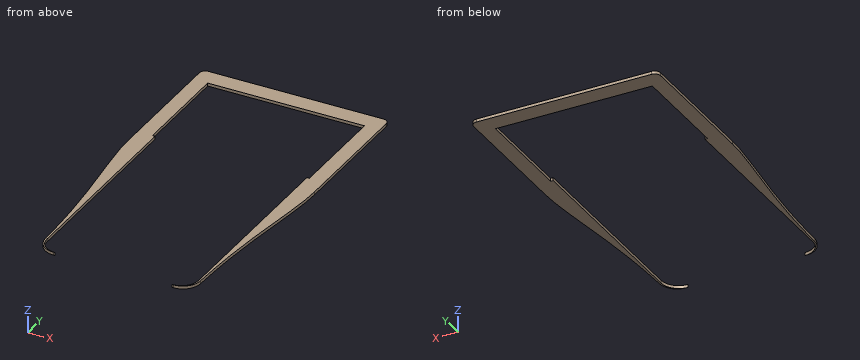
```python
from build123d import *

# Parameters (mm, degrees)
BOSS_EXTRUDE1_START = -1.5
BOSS_EXTRUDE1_DEPTH = 1.5
CUT_EXTRUDE1_DEPTH  = 14
FILLET1_R           = 8.7
FILLET2_R           = 3


# Read off the part's stored shape, not the designer's step: Boss-Extrude1
with BuildPart() as part:
    # Boss-Extrude1 outline → Boss-Extrude1 (new body)
    with BuildSketch(Plane.XY.offset(BOSS_EXTRUDE1_START)):
        with BuildLine():
            Line((101.710048323, 103.170955585), (101.710048323, 33.070955585))
            add(Edge.make_bspline(
                [(101.710048323, 33.070955585), (101.710048323, 14.099715191), (109.710048323, -16.929044415), (109.710048323, -66.929044415)],
                knots=[0, 0, 0, 0, 1, 1, 1, 1], degree=3))
            Line((109.710048323, -66.929044415), (187.010048323, -66.929044415))
            add(Edge.make_bspline(
                [(195.010048323, 33.070955585), (195.010048323, 11.335097122), (187.010048323, -16.929044415), (187.010048323, -66.929044415)],
                knots=[0, 0, 0, 0, 1, 1, 1, 1], degree=3))
            Line((195.010048323, 33.070955585), (195.010048323, 103.170955585))
            Line((195.010048323, 103.170955585), (101.710048323, 103.170955585))
        make_face()
    extrude(amount=BOSS_EXTRUDE1_DEPTH)

    # Sketch2 → Cut-Extrude1 (cut)
    with BuildSketch(Plane.XY):
        with BuildLine():
            Line((109.160048323, 94.070955585), (187.460048323, 94.070955585))
            Line((187.460048323, 94.070955585), (187.460048323, 42.570955585))
            Line((187.460048323, 42.570955585), (186.260048323, 42.570955585))
            Line((186.260048323, 42.570955585), (186.260048323, -58.229044415))
            ThreePointArc((186.260048323, -58.229044415), (183.711877319, -64.380873411), (177.560048323, -66.929044415))
            Line((177.560048323, -66.929044415), (119.160048323, -66.929044415))
            ThreePointArc((119.160048323, -66.929044415), (113.008219327, -64.380873411), (110.460048323, -58.229044415))
            Line((110.460048323, -58.229044415), (110.460048323, 42.570955585))
            Line((110.460048323, 42.570955585), (109.160048323, 42.570955585))
            Line((109.160048323, 42.570955585), (109.160048323, 94.070955585))
        make_face()
    extrude(amount=-CUT_EXTRUDE1_DEPTH, mode=Mode.SUBTRACT)

    # Fillet1
    fillet1_edges = [part.edges().sort_by_distance(p)[0] for p in [
        (187.010048323, -66.929044415, -0.75),
        (109.710048323, -66.929044415, -0.75),
    ]]
    fillet(fillet1_edges, radius=FILLET1_R)

    # Fillet2
    fillet2_edges = [part.edges().sort_by_distance(p)[0] for p in [
        (101.710048323, 103.170955585, -0.75),
        (195.010048323, 103.170955585, -0.75),
    ]]
    fillet(fillet2_edges, radius=FILLET2_R)


solid = part.part
```
Could you check a few things on this model? Use its own coordinates, in mm. Give positions to 0.01 mm unless a question says otherwise; leave off trailing zeros. Order: outer loops, then holes, each group sorted by start corner. A loop starts at its lowest first (then second) coordinate and runs counter-clockwise, first axis right, second up.
Q1. I'm going to push a flat-ended pin straight in: P1, Ø0.8, axis at y = 0.5, z = -0.5, coming from the -X side. Where does the tip first touch, or does it pass through?
Q2. Suppose I cut it at C-C, the plane x = 136. Write out the boundary of the cut face in (y, z), and give its area (4 significant figures).
Q3. Suppose I cut it at B-B, the plane y = 65.5. Write out the boundary of the cut face in (x, z).
Q4. If I drill on line 1 along X through (y, z) = (47, -0.95); line 2 along Y through (x, z) = (142, -1.15); line 3 along X through (y, z) = (38, -1.05), over which ranges is the centre line in solid material (lowest first)?
Q5. Suppose I cut it at A-A, the plane y = 39.5. Write out the boundary of the cut face in (x, z), and give its area (4 significant figures).
Solution:
1. P1: stops at x = 104.93
2. outline: (94.07, -1.5) - (103.17, -1.5) - (103.17, 0) - (94.07, 0) - close
2. area: 13.65 mm2
3. outline: (101.71, -1.5) - (109.16, -1.5) - (109.16, 0) - (101.71, 0) - close; (187.46, -1.5) - (195.01, -1.5) - (195.01, 0) - (187.46, 0) - close
4. line 1: x = 101.71 to 109.16, 187.46 to 195.01
4. line 2: y = 94.07 to 103.17
4. line 3: x = 101.71 to 110.46, 186.26 to 195.01
5. outline: (101.71, -1.5) - (110.46, -1.5) - (110.46, 0) - (101.71, 0) - close; (186.26, -1.5) - (195.01, -1.5) - (195.01, 0) - (186.26, 0) - close
5. area: 26.25 mm2
